The listing builds one solid part. Answer for the finished solid, in the listing's coordinates (mm). Face numbers are marked on the shaded views. A direction names the side the tool comes from. Coordinates: 2 decimals unless noted, no trailing zeros. Write each loop counter-clockwise with the first axis right and the second up, starting at its lowest first coordinate (ties: lowest second). Pieces come first, ordered by that corner, then holes.
(1) Which of the six approach directions +Z, -Z, +X, -X, +Y, -Y give full straight-line access (tool end or side, diameter ignored) to the marked faces 5 and 6?
(2) The part is cut by section A-A on z = 1. Determine the outline of the cut face in (x, y).
(3) The part is cut by section C-C on x = -2. Determine the outline of the cut face in (y, z).
(4) Straight lines are drawn through the part: line 1 (Y direction, x = -6, z = 0.75); line 2 (X direction, y = -1.75, z = 1.75); line 3 (Y direction, x = 0, z = 0.45). For each, find the intervals that lie inside material, in ascending order.
(5) Given P1, Ø5, axis at x = -6, y = -2, coming from the +Z side; P2, Ø2, axis at x = 0.5, y = 4.5, coming from the -Z side, each flat-ended and moving along its own axis, determine where each tip first touches the part or whether it passes through.
(6) For a pull along Y with two mould halves and no side action, classify the marked faces 1, 2, 3 and 4 as +Y half, -Y half, draft (parallel to the pull), parting line (faces both ways), or undercut.
(7) The part is cut by section B-B on x = -6. Determine the outline of the cut face in (y, z).
(8) The part is cut by section D-D on y = 4.75. Determine the outline of the cut face in (x, z).
from build123d import *

# Parameters (mm, degrees)
SKETCH1_W            = 20
SKETCH1_H            = 12
BOSS_EXTRUDE1_DEPTH  = 3
SKETCH2_W            = 20
SKETCH2_H            = 4
CUT_EXTRUDE1_DEPTH   = 0.5
M3_CLEARANCE_HOLE1_D = 3.2


with BuildPart() as part:
    # Sketch1 → Boss-Extrude1 (new body)
    with BuildSketch(Plane.XY):
        Rectangle(SKETCH1_W, SKETCH1_H)
    extrude(amount=BOSS_EXTRUDE1_DEPTH)

    # Sketch2 → Cut-Extrude1 (cut)
    with BuildSketch(Plane(origin=(0, 0, 0), x_dir=(-1, 0, 0), z_dir=(0, 0, -1))):
        with Locations((0, 4)):
            Rectangle(SKETCH2_W, SKETCH2_H)
    extrude(amount=-CUT_EXTRUDE1_DEPTH, mode=Mode.SUBTRACT)

    # M3 Clearance Hole1 (through all)
    with Locations(Plane.XY.offset(3)):
        with Locations((-6, -2), (6, -2)):
            Hole(M3_CLEARANCE_HOLE1_D / 2)


solid = part.part
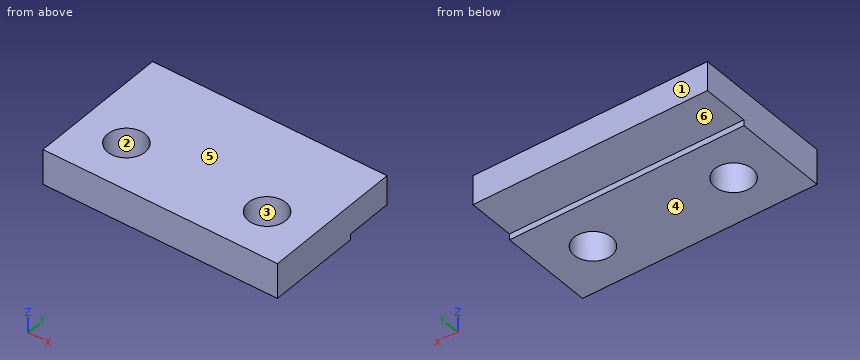
Model answer:
1. face 5: +Z, +X, -X, +Y, -Y
1. face 6: -Z, +X, -X, +Y
2. outline: (-10, -6) - (10, -6) - (10, 6) - (-10, 6) - close; hole circle Ø3.2 at (-6, -2); hole circle Ø3.2 at (6, -2)
3. outline: (-6, 0) - (2, 0) - (2, 0.5) - (6, 0.5) - (6, 3) - (-6, 3) - close
4. line 1: y = -6 to -3.6, -0.4 to 6
4. line 2: x = -10 to -7.58, -4.42 to 4.42, 7.58 to 10
4. line 3: y = -6 to 2
5. P1: stops at z = 3
5. P2: stops at z = 0.5
6. face 1: +Y half
6. face 2: undercut
6. face 3: undercut
6. face 4: draft
7. outline: (-6, 0) - (-3.6, 0) - (-3.6, 3) - (-6, 3) - close; (-0.4, 0) - (2, 0) - (2, 0.5) - (6, 0.5) - (6, 3) - (-0.4, 3) - close
8. outline: (-10, 0.5) - (10, 0.5) - (10, 3) - (-10, 3) - close
